Could you check a few things on this model? Use its own coordinates, in mm. A direction names the side the tool comes from. Give positions to 0.01 mm unless a question says otherwise; leave off trailing zeros. Order: outer loops, then holes, each group sorted by start corner. A loop starts at its lowest first (then second) coordinate and runs counter-clockwise, first axis right, second up. Notation, with made-up numbers: (-11.5, 62) -> (41.5, 62) arc R18 cw to (41.5, 91) -> close; hole circle Ø1 at (57.5, 14.25). An arc over 180 degrees is marked (long way). Use one line per item in the form item = value. Start each with the question number.
from build123d import *

# Parameters (mm, degrees)
SKETCH1_R           = 11.495405
BOSS_EXTRUDE2_DEPTH = 4.7625
SKETCH1_4_R         = 11.495405
BOSS_EXTRUDE3_DEPTH = 3.175
FILLET1_R           = 3.175
CHAMFER1_SIZE       = 0.889


with BuildPart() as part:
    # Sketch1 → Boss-Extrude2 (new, symmetric)
    with BuildSketch(Plane.XY):
        with BuildLine():
            ThreePointArc((14.43672871, 2.668051275), (-5.197044393, 13.730563099), (-12.585193267, -7.559797873))
            ThreePointArc((-12.585193267, -7.559797873), (5.197044393, -13.730563099), (14.43672871, 2.668051275))
        make_face()
        with Locations(Location((0, 0, 0), (0, 0, 180))):
            Circle(SKETCH1_R, mode=Mode.SUBTRACT)
    extrude(amount=BOSS_EXTRUDE2_DEPTH, both=True)

    # Sketch1_4 → Boss-Extrude3 (add, symmetric)
    # profile 1 of 2: a face of its own
    with BuildSketch(Plane.XY):
        with BuildLine():
            ThreePointArc((-12.585193267, -7.559797873), (-10.89585042, -11.492870345), (-10.31875, -15.734319794))
            Line((-10.31875, -15.734319794), (-10.31875, -46.214319794))
            Line((-10.31875, -46.214319794), (10.31875, -46.214319794))
            Line((10.31875, -46.214319794), (10.31875, -27.262081536))
            Line((10.31875, -27.262081536), (24.759911139, -43.605812684))
            Line((24.759911139, -43.605812684), (40.225193096, -29.940840667))
            Line((40.225193096, -29.940840667), (18.15100753, -4.958462121))
            ThreePointArc((18.15100753, -4.958462121), (15.775028495, -1.397891668), (14.43672871, 2.668051275))
            ThreePointArc((14.43672871, 2.668051275), (5.197044393, -13.730563099), (-12.585193267, -7.559797873))
        make_face()
        with BuildLine():
            ThreePointArc((5.55625, -35.895569794), (0, -41.451819794), (-5.55625, -35.895569794))
            Line((-5.55625, -35.895569794), (-5.55625, -31.133069794))
            ThreePointArc((-5.55625, -31.133069794), (0, -25.576819794), (5.55625, -31.133069794))
            Line((5.55625, -31.133069794), (5.55625, -35.895569794))
        make_face(mode=Mode.SUBTRACT)
        with BuildLine():
            ThreePointArc((29.823795866, -25.361654769), (29.339097036, -33.204415455), (21.496336351, -32.719716625))
            Line((21.496336351, -32.719716625), (18.34288127, -29.150805404))
            ThreePointArc((18.34288127, -29.150805404), (18.8275801, -21.308044718), (26.670340785, -21.792743548))
            Line((26.670340785, -21.792743548), (29.823795866, -25.361654769))
        make_face(mode=Mode.SUBTRACT)
    # profile 2 of 2: a face of its own
    with BuildSketch(Plane.XY):
        with BuildLine():
            ThreePointArc((14.43672871, 2.668051275), (-5.197044393, 13.730563099), (-12.585193267, -7.559797873))
            ThreePointArc((-12.585193267, -7.559797873), (5.197044393, -13.730563099), (14.43672871, 2.668051275))
        make_face()
        with Locations(Location((0, 0, 0), (0, 0, 180))):
            Circle(SKETCH1_4_R, mode=Mode.SUBTRACT)
    extrude(amount=BOSS_EXTRUDE3_DEPTH, both=True)

    # Fillet1
    fillet1_edges = [part.edges().sort_by_distance(p)[0] for p in [
        (-10.31875, -46.214319794, 0),
        (10.31875, -46.214319794, 0),
        (10.31875, -27.262081536, 0),
        (24.759911139, -43.605812684, 0),
        (40.225193096, -29.940840667, 0),
    ]]
    fillet(fillet1_edges, radius=FILLET1_R)

    # Chamfer1
    chamfer1_edges = [part.edges().sort_by_distance(p)[0] for p in [
        (11.495405, 0, -4.7625),
        (11.495405, 0, 4.7625),
    ]]
    chamfer(chamfer1_edges, length=CHAMFER1_SIZE)


solid = part.part
(1) Imagine slicing it at A-A (x = 0). Write out the boundary of the cut face in (y, z) (1 decimal), plus the area to 3 significant figures.
(2) We'd pull the mould along X, two halves only. Please class faces 1 (the cylindrical face through (15.8, -1.45, 0.04)), 2 (the cylindrical face through (-10.912, -11.435, 0.044)), 3 (the flat face through (-5.556, -34, 0)): pulls with the +X half, pulls with the -X half, needs draft (parallel to the pull), parting line crosses it, or undercut.
(3) Please list where these lines run through material, in increasing order: probe 1 along X at (y, z) = (-27, 1.25); probe 2 along Y at (x, z) = (0, 1.25); probe 3 along X at (y, z) = (-28, -2.5).
(4) Imagine slicing it at B-B (y = 0). Write out the boundary of the cut face in (x, z) (1 decimal).
(5) Imagine slicing it at D-D (x = 25.5). Write out the boundary of the cut face in (y, z) (3 decimals), plus the area to 3 significant figures.
(6) Imagine slicing it at C-C (z = 1). Give the number of separate pieces and of enclosed holes in the cut face, plus the area to 3 significant figures.
(7) Which directions (+Z, -Z, +X, -X, +Y, -Y) give clear straight access to the entire face, cutting with the end or side of a thin tool? Please do faces 4 (the flat face through (-8, -10, -4.762)), 5 (the flat face through (19.218, -37.334, -0.044)), 6 (the flat face through (19.94, -30.96, 0.04)).
(8) I'm going to push flat-ended pins straight in: pin 1 Ø4 at (y, z) = (-19.5, 0) entering from +X; pin 2 Ø3 at (x, y) = (19, -10) entering from +Z (3 decimals); pin 3 Ø20.5 at (x, y) = (0, 0) entering from -Z; pin 4 Ø2 at (y, z) = (-30.5, 0) entering from -X. Where does each tip first touch, or does it pass through?
Calculated:
q1.outline = (-46.2, -3.2) -> (-41.5, -3.2) -> (-41.5, 3.2) -> (-46.2, 3.2) -> close; (-25.6, -3.2) -> (-14.7, -3.2) -> (-14.7, -4.8) -> (-12.4, -4.8) -> (-11.5, -3.9) -> (-11.5, 3.9) -> (-12.4, 4.8) -> (-14.7, 4.8) -> (-14.7, 3.2) -> (-25.6, 3.2) -> close; (11.5, -3.9) -> (12.4, -4.8) -> (14.7, -4.8) -> (14.7, 4.8) -> (12.4, 4.8) -> (11.5, 3.9) -> close
q1.area = 159 mm2
q2.face_1 = pulls with the +X half
q2.face_2 = pulls with the -X half
q2.face_3 = undercut
q3.probe_1 = -10.32 to -3.71, 3.71 to 17.16, 30.83 to 37.63
q3.probe_2 = -46.21 to -41.45, -25.58 to -11.5, 11.5 to 14.68
q3.probe_3 = -10.32 to -4.59, 4.59 to 17.56, 31.12 to 38.45
q4.outline = (-14.7, -4.8) -> (-12.4, -4.8) -> (-11.5, -3.9) -> (-11.5, 3.9) -> (-12.4, 4.8) -> (-14.7, 4.8) -> close; (11.5, -3.9) -> (12.4, -4.8) -> (14.7, -4.8) -> (14.7, -3.2) -> (15.2, -3.2) -> (15.2, 3.2) -> (14.7, 3.2) -> (14.7, 4.8) -> (12.4, 4.8) -> (11.5, 3.9) -> close
q5.outline = (-42.265, -3.175) -> (-34.595, -3.175) -> (-34.595, 3.175) -> (-42.265, 3.175) -> close; (-20.791, -3.175) -> (-13.276, -3.175) -> (-13.276, 3.175) -> (-20.791, 3.175) -> close
q5.area = 96.4 mm2
q6.separate_pieces = 1
q6.enclosed_holes = 3
q6.area = 1,300 mm2
q7.face_4 = -Z, +X, -X, +Y, -Y
q7.face_5 = +Z, -Z, -Y
q7.face_6 = +Z, -Z
q8.pin_1 = 32.77
q8.pin_2 = 3.175
q8.pin_3 = through
q8.pin_4 = -10.32
